```python
from build123d import *

# Parameters (mm, degrees)
SKETCH_W            = 27
SKETCH_H            = 20
PAD_DEPTH           = 3
PAD001_DEPTH        = 3
LINEARPATTERN_COUNT = 3
LINEARPATTERN_PITCH = 6
FILLET_R            = 9


with BuildPart() as part:
    # Sketch → Pad (new body)
    with BuildSketch(Plane.XY):
        Rectangle(SKETCH_W, SKETCH_H)
    extrude(amount=PAD_DEPTH)

    # Sketch001 → Pad001 (new body)
    with BuildSketch(Plane.YZ.offset(13.5)):
        Polygon((-6.9, 3), (-5, 3), (-4, 0), (-7.9, 0), align=None)
    pad001 = extrude(amount=PAD001_DEPTH)

    # LinearPattern: Pad001 ×3
    with Locations(*[(0, i * LINEARPATTERN_PITCH, 0) for i in range(1, LINEARPATTERN_COUNT)]):
        add(pad001)

    # Fillet
    fillet_edges = [part.edges().sort_by_distance(p)[0] for p in [
        (-13.5, 10, 1.5),
        (-13.5, -10, 1.5),
    ]]
    fillet(fillet_edges, radius=FILLET_R)


solid = part.part
```
Geometry: final body of the model. Coordinates: model frame, mm. A direction names the side the tool comes from. Round coordinates to 2 decimals unless told otherwise and drop trailing zeros. Order: outer loops, then holes, each group sorted by start corner. A loop starts at its lowest first (then second) coordinate and runs counter-clockwise, first axis right, second up. Notation, with made-up numbers: M -40,12.25 L 19,12.25 A7 cw 19,21.25 Z; hole C 46.25,82.5 d4. An arc over 180 degrees is marked long. Use one line per item in the form item = value. Start each with the question number.
Q1. Pin query (flat end, axial travel): pin 1 Ø1.5 at (x, z) = (-8, 1.5) entering from -Y; pin 2 Ø1.5 at (y, z) = (2.5, 2) entering from +X. Return the tip coordinate at first contact, or that it passes through.
Q2. Cut plane C-C (z = 0.55). Return loops of the section in (x, y), and give its area (3 significant figures).
Q3. Cut plane A-A (z = 2.4). Return loops of the section in (x, y), and give its area (3 significant figures).
Q4. Access query for faces 4 (the face through (1, 0, 0)), 5 (the face through (13.5, -3, 2)), 6 (the face through (-13.5, 0, 1)), 7 (the face through (15, 7.5, 1.5)), 8 (the face through (13.5, -9, 1)). Directions: +Z, -Z, +X, -X, +Y, -Y. A direction counts if a zero-diameter tool reaches every point of the face in a straight line with its end or side. Return the directions, or none.
Q5. Cut plane D-D (x = -10.25). Return loops of the section in (y, z), and give its area (3 significant figures).
Q6. Cut plane B-B (y = 4.75). Return loops of the section in (x, z), and give its area (3 significant figures).
Q7. Mould query, pull axis Y, two halves, no side actions, for faces 1 (the face through (13.5, 9, 1)), 2 (the face through (-10.934, 7.294, 1.521)), 3 (the face through (13.5, 3, 2)). Classes: +Y half, -Y half, draft (parallel to the pull), parting line (faces both ways), or undercut.
Q8. Material intervals for line 1 (Y direction, x = -9, z = 2.1); line 2 (X direction, y = -2.25, z = 2.85); line 3 (X direction, y = -6.75, z = 0.2), sorted ascending. Write a range as [from, to].
Geometry results:
q1.pin_1 = -9.57
q1.pin_2 = 13.5
q2.outline = M -13.5,-1 A9 ccw -4.5,-10 L 13.5,-10 L 13.5,-7.72 L 16.5,-7.72 L 16.5,-4.18 L 13.5,-4.18 L 13.5,-1.72 L 16.5,-1.72 L 16.5,1.82 L 13.5,1.82 L 13.5,4.28 L 16.5,4.28 L 16.5,7.82 L 13.5,7.82 L 13.5,10 L -4.5,10 A9 ccw -13.5,1 Z
q2.area = 537 mm^2
q3.outline = M -13.5,-1 A9 ccw -4.5,-10 L 13.5,-10 L 13.5,-7.1 L 16.5,-7.1 L 16.5,-4.8 L 13.5,-4.8 L 13.5,-1.1 L 16.5,-1.1 L 16.5,1.2 L 13.5,1.2 L 13.5,4.9 L 16.5,4.9 L 16.5,7.2 L 13.5,7.2 L 13.5,10 L -4.5,10 A9 ccw -13.5,1 Z
q3.area = 526 mm^2
q4.face_4 = -Z, +X, -X, +Y, -Y
q4.face_5 = +Z, +X
q4.face_6 = +Z, -Z, -X, +Y, -Y
q4.face_7 = +Z, +X, +Y
q4.face_8 = +Z, +X, -Y
q5.outline = M -7.92,0 L 7.92,0 L 7.92,3 L -7.92,3 Z
q5.area = 47.5 mm^2
q6.outline = M -12.68,0 L 16.5,0 L 16.5,1.95 L 13.5,1.95 L 13.5,3 L -12.68,3 Z
q6.area = 84.4 mm^2
q7.face_1 = draft
q7.face_2 = +Y half
q7.face_3 = undercut
q8.line_1 = [-8.79, 8.79]
q8.line_2 = [-13.41, 13.5]
q8.line_3 = [-11.42, 16.5]
